```python
from build123d import *

# Parameters (mm, degrees)
F0_R     = 1.6
F1_DEPTH = 1.5


with BuildPart() as f1:
    # F0 (on Top) → F1 (new body)
    with BuildSketch(Plane.XY):
        with BuildLine():
            Line((-43.070649, 22.894378), (-58.070649, 22.894378))
            ThreePointArc((-58.070649, 22.894378), (-61.606183, 21.429912), (-63.070649, 17.894378))
            ThreePointArc((-63.070649, 17.894378), (-61.606183, 14.358844), (-58.070649, 12.894378))
            Line((-58.070649, 12.894378), (-53.070649, 12.894378))
            Line((-53.070649, 12.894378), (-43.070649, 12.894378))
            Line((-43.070649, 12.894378), (-43.070649, 22.894378))
        make_face()
        with Locations((-58.070649, 17.894378)):
            Circle(F0_R, mode=Mode.SUBTRACT)
        with Locations((-48.070649, 17.894378)):
            Circle(F0_R, mode=Mode.SUBTRACT)
        with BuildLine():
            Line((-43.070649, -2.105622), (-43.070649, 12.894378))
            Line((-43.070649, 12.894378), (-53.070649, 12.894378))
            Line((-53.070649, 12.894378), (-53.070649, -2.105622))
            ThreePointArc((-53.070649, -2.105622), (-51.606183, -5.641156), (-48.070649, -7.105622))
            ThreePointArc((-48.070649, -7.105622), (-44.535115, -5.641156), (-43.070649, -2.105622))
        make_face()
        with Locations((-48.070649, -2.105622)):
            Circle(F0_R, mode=Mode.SUBTRACT)
        with Locations((-48.070649, 7.894378)):
            Circle(F0_R, mode=Mode.SUBTRACT)
    extrude(amount=F1_DEPTH)


solid = f1.part
```
CAD build for the part. Positions are in the model's coordinates, mm. A direction names the side the tool comes from. Round coordinates to 2 decimals unless told otherwise and drop trailing zeros. Order: outer loops, then holes, each group sorted by start corner. A loop starts at its lowest first (then second) coordinate and runs counter-clockwise, first axis right, second up. Notation, with made-up numbers: (25, 1.5) -> (79, 1.5) arc R32 ccw to (79, 36.5) -> close; hole circle Ø1 at (1, -11). An arc over 180 degrees is marked (long way). Write item = value, one per line.
(1) Cut at D-D (y = 6). Write the cut outline in (x, z), plus the area to 3 significant figures.
Answers follow:
outline = (-53.07, 0) -> (-43.07, 0) -> (-43.07, 1.5) -> (-53.07, 1.5) -> close
area = 15.0 mm²
(2) Pull direction Y, two halves, no side cores. Call faces 1 (the flat face through (-51, 11, 1.5)), 2 (the flat face through (-50, 22.894, 1)), 3 (the cylindrical face through (-46.545, -1.625, 0.74)): +Y half, -Y half, draft (parallel to the pull), parting line (faces both ways), or undercut.
Answers follow:
face_1 = draft
face_2 = +Y half
face_3 = undercut
(3) Cut at A-A (x = -47). Write the cut outline in (y, z).
Answers follow:
outline = (-6.99, 0) -> (-3.29, 0) -> (-3.29, 1.5) -> (-6.99, 1.5) -> close; (-0.92, 0) -> (6.71, 0) -> (6.71, 1.5) -> (-0.92, 1.5) -> close; (9.08, 0) -> (16.71, 0) -> (16.71, 1.5) -> (9.08, 1.5) -> close; (19.08, 0) -> (22.89, 0) -> (22.89, 1.5) -> (19.08, 1.5) -> close
(4) Flat gauge pins, fed straight in: P1, Ø2.5, axis at x = -48.07, y = 7.89, coming from the -Z side; P2, Ø0.8, axis at x = -55, z = 1, coming from the -Y side; P3, Ø0.8, axis at y = 8.5, z = 1, coming from the -X side. Where does each tip first touch, or does it go through?
Answers follow:
P1 = through
P2 = 12.89
P3 = -53.07
(5) Cut at C-C (z = 0.4). Write the cut outline in (x, y).
Answers follow:
outline = (-58.07, 12.89) -> (-53.07, 12.89) -> (-53.07, -2.11) arc R5 ccw to (-43.07, -2.11) -> (-43.07, 22.89) -> (-58.07, 22.89) arc R5 ccw to start; hole circle Ø3.2 at (-58.07, 17.89); hole circle Ø3.2 at (-48.07, -2.11); hole circle Ø3.2 at (-48.07, 7.89); hole circle Ø3.2 at (-48.07, 17.89)
(6) Cut at B-B (x = -57.75). Write the cut outline in (y, z), plus the area to 3 significant figures.
Answers follow:
outline = (12.89, 0) -> (16.33, 0) -> (16.33, 1.5) -> (12.89, 1.5) -> close; (19.46, 0) -> (22.89, 0) -> (22.89, 1.5) -> (19.46, 1.5) -> close
area = 10.3 mm²
(7) Drill centre lines: L1, parallel to Y at x = -49.5, z = 0.1; L2, parallel to X at y = 16.5, z = 1.35; L3, parallel to Y at x = -58.75, z = 1.2. Where is each one in solid material? Low to high.
Answers follow:
L1 = -6.9 to -2.82, -1.39 to 7.18, 8.61 to 17.18, 18.61 to 22.89
L2 = -62.87 to -58.86, -57.29 to -48.86, -47.29 to -43.07
L3 = 12.94 to 16.45, 19.34 to 22.85
(8) 3-axis set-ups, long thin cutter, end or side, ignore diameter. For faces 4 (the flat face through (-43.071, 10, 1)), 5 (the flat face through (-56, 12.894, 1)): which of +Z, -Z, +X, -X, +Y, -Y reach the whole face in a straight line?
Answers follow:
face_4 = +Z, -Z, +X, +Y, -Y
face_5 = +Z, -Z, -X, -Y
